```python
from build123d import *

# Parameters (mm, degrees)
F0_W     = 101.6
F0_H     = 127
F1_DEPTH = 3.175
F2_R     = 2.263003
F3_DEPTH = 3.176
F4_R     = 3.175
F5_DEPTH = 3.176


with BuildPart() as f1:
    # F0 (on Front) → F1 (new body)
    with BuildSketch(Plane.XZ):
        with Locations((-50.659383, 43.110808)):
            Rectangle(F0_W, F0_H)
    extrude(amount=F1_DEPTH)

    # F2 (on face) → F3 (cut, through all)
    with BuildSketch(Plane.XZ.offset(3.175)):
        with Locations((-50.659383, 79.876246)):
            Circle(F2_R)
        with Locations((-50.659383, 14.293446)):
            Circle(F2_R)
    extrude(amount=-F3_DEPTH, mode=Mode.SUBTRACT)

    # F4 (on face) → F5 (cut, through all)
    with BuildSketch(Plane.XZ.offset(3.175)):
        with Locations((-92.782468, 59.784846)):
            Circle(F4_R)
        with Locations((-92.782468, 34.384846)):
            Circle(F4_R)
        with Locations((-8.536297, 34.384846)):
            Circle(F4_R)
        with Locations((-8.536297, 59.784846)):
            Circle(F4_R)
    extrude(amount=-F5_DEPTH, mode=Mode.SUBTRACT)


solid = f1.part
```
For this review, take the finished solid that the model builds, in its own axes (mm). Give positions to 0.01 mm unless a question says otherwise; leave off trailing zeros. Loops run counter-clockwise (first coordinate to the right, second up) from the corner with the lowest first, then second, coordinate; pieces in that order, holes last. Notation, with made-up numbers: M 20,9.5 L 66,9.5 A13 cw 66,21.5 Z; hole C 20,13.25 d3. An arc over 180 degrees is marked long. One line per item, written item: value. Start each with the question number.
Q1. Add section A-A (x = -7.5). Give the boundary of the cut face in (y, z) (3 decimals).
Q2. Draft analysis for pull direction X (two halves, no side actions). For faces 1 (the face through (0.141, -2, 42)), 2 (the face through (-49.443, -1.61, 81.784)), 3 (the face through (-51, -3.175, 44)), state which applies: released by +X, released by -X, zero draft, split by the parting line, or undercut.
Q3. For L1, parallel to X at y = -1.35, z = 36; L2, parallel to Z at x = -93.5, y = -2; L3, parallel to Z at x = -94, y = -2.6, list the stretches that pass through material, from the lowest coordinate up.
Reply:
1. outline: M -3.175,-20.389 L 0,-20.389 L 0,31.384 L -3.175,31.384 Z; M -3.175,37.386 L 0,37.386 L 0,56.784 L -3.175,56.784 Z; M -3.175,62.786 L 0,62.786 L 0,106.611 L -3.175,106.611 Z
2. face 1: released by +X
2. face 2: undercut
2. face 3: zero draft
3. L1: -101.46 to -95.52, -90.05 to -11.27, -5.8 to 0.14
3. L2: -20.39 to 31.29, 37.48 to 56.69, 62.88 to 106.61
3. L3: -20.39 to 31.45, 37.32 to 56.85, 62.72 to 106.61
